```python
from build123d import *

# Parameters (mm, degrees)
BOSS_EXTRUDE1_DEPTH = 44.704
CUT_EXTRUDE1_DEPTH  = 55.481223747
CUT_EXTRUDE2_DEPTH  = 55.481223747


with BuildPart() as part:
    # Sketch1 → Boss-Extrude1 (new body)
    with BuildSketch(Plane(origin=(0, 0, 0), x_dir=(1, 0, 0), z_dir=(0, 1, 0))):
        with BuildLine():
            Line((19.604538786, -1.778), (-19.604538786, -1.778))
            ThreePointArc((-19.604538786, -1.778), (0, -19.685), (19.604538786, -1.778))
        make_face()
        with BuildLine():
            Line((-24.13, 1.778), (-24.13, -1.778))
            Line((-24.13, -1.778), (-19.604538786, -1.778))
            ThreePointArc((-19.604538786, -1.778), (-19.685, 0), (-19.604538786, 1.778))
            Line((-19.604538786, 1.778), (-24.13, 1.778))
        make_face()
        with BuildLine():
            ThreePointArc((19.685, 0), (19.664874408, -0.889909828), (19.604538786, -1.778))
            Line((19.604538786, -1.778), (24.13, -1.778))
            Line((24.13, -1.778), (24.13, 1.778))
            Line((24.13, 1.778), (19.604538786, 1.778))
            ThreePointArc((19.604538786, 1.778), (19.664874408, 0.889909828), (19.685, 0))
        make_face()
        with BuildLine():
            ThreePointArc((-19.604538786, 1.778), (-19.685, 0), (-19.604538786, -1.778))
            Line((-19.604538786, -1.778), (19.604538786, -1.778))
            ThreePointArc((19.604538786, -1.778), (19.664874408, -0.889909828), (19.685, 0))
            ThreePointArc((19.685, 0), (19.664874408, 0.889909828), (19.604538786, 1.778))
            Line((19.604538786, 1.778), (-19.604538786, 1.778))
        make_face()
        with BuildLine():
            ThreePointArc((-10.145068686, 16.869404446), (-16.679250829, 10.454750919), (-19.604538786, 1.778))
            Line((-19.604538786, 1.778), (19.604538786, 1.778))
            ThreePointArc((19.604538786, 1.778), (16.371852187, 10.929852742), (9.158931314, 17.424500056))
            Line((9.158931314, 17.424500056), (9.158931314, 11.559229776))
            Line((9.158931314, 11.559229776), (-10.145068686, 11.559229776))
            Line((-10.145068686, 11.559229776), (-10.145068686, 16.869404446))
        make_face()
    extrude(amount=BOSS_EXTRUDE1_DEPTH)

    # Sketch3 → Cut-Extrude1 (cut, through all)
    with BuildSketch(Plane(origin=(0, 44.704, 0), x_dir=(1, 0, 0), z_dir=(0, 1, 0))):
        with BuildLine():
            Line((-18.40799177, 0.508), (-18.40799177, -0.508))
            ThreePointArc((-18.40799177, -0.508), (0, -18.415), (18.40799177, -0.508))
            Line((18.40799177, -0.508), (18.40799177, 0.508))
            ThreePointArc((18.40799177, 0.508), (16.176802096, 8.799051026), (10.428931314, 15.177273031))
            Line((10.428931314, 15.177273031), (10.428931314, 10.289229776))
            Line((10.428931314, 10.289229776), (-11.415068686, 10.289229776))
            Line((-11.415068686, 10.289229776), (-11.415068686, 14.450205254))
            ThreePointArc((-11.415068686, 14.450205254), (-16.460559091, 8.256041389), (-18.40799177, 0.508))
        make_face()
    extrude(amount=-CUT_EXTRUDE1_DEPTH, mode=Mode.SUBTRACT)

    # Sketch4 → Cut-Extrude2 (cut, through all)
    with BuildSketch(Plane(origin=(0, 44.704, 0), x_dir=(1, 0, 0), z_dir=(0, 1, 0))):
        Polygon((-11.415068686, 14.450205254), (-10.145068686, 15.334289128), (9.158931314, 15.334289128), (10.428931314, 15.177273031), (10.428931314, 10.289229776), (-11.415068686, 10.289229776), align=None)
    extrude(amount=-CUT_EXTRUDE2_DEPTH, mode=Mode.SUBTRACT)


solid = part.part
```
Input: part model. Units: mm. Frame: model coordinates. A direction names the side the tool comes from. Give positions to 0.01 mm unless a question says otherwise; leave off trailing zeros. Order: outer loops, then holes, each group sorted by start corner. A loop starts at its lowest first (then second) coordinate and runs counter-clockwise, first axis right, second up. Notation, with made-up numbers: (7, -34.5) - (12, -34.5) arc R30 ccw to (12, -5.5) - close; hole circle Ø4 at (45.25, 41.5). An arc over 180 degrees is marked (long way). One line per item, written item: value.
1. Draft query along Z for faces 1 (the face through (0, 44.704, 19)), 2 (the face through (22, 22, -1.778)), 3 (the face through (-10.789, 22.665, -14.886)), 4 (the face through (-16.41, 22.66, -8.36)). Return one class per face: released by +Z, released by -Z, zero draft, split by the parting line, or undercut.
Determined:
face 1: zero draft
face 2: released by -Z
face 3: undercut
face 4: undercut
2. Pin query (flat end, axial travel): pin 1 Ø2.5 at (x, y) = (-21, 33.5) entering from -Z; pin 2 Ø2.5 at (x, y) = (22, 21) entering from +Z; pin 3 Ø1.7 at (y, z) = (19, -16) entering from +X. Return the tip coordinate at first contact, or that it passes through.
Determined:
pin 1: z = -1.78
pin 2: z = 1.78
pin 3: x = 12.57
3. Cut plane D-D, the plane x = 0. Output: boundary loops of the cut face in (y, z) (3 decimals), and give its area (3 significant figures).
Determined:
outline: (0, 18.415) - (44.704, 18.415) - (44.704, 19.685) - (0, 19.685) - close
area: 56.8 mm2
4. Cut plane A-A, the plane z = 5.5. Output: boundary loops of the cut face in (x, y), and give its area (3 significant figures).
Determined:
outline: (-18.9, 0) - (-17.57, 0) - (-17.57, 44.7) - (-18.9, 44.7) - close; (17.57, 0) - (18.9, 0) - (18.9, 44.7) - (17.57, 44.7) - close
area: 119 mm2
5. Line query: probe 1 along X at (y, z) = (34.5, 0); probe 2 along Z at (x, y) = (-10.5, 42); probe 3 along Z at (x, y) = (20.5, 29). Output: solid intervals per line, ascending.
Determined:
probe 1: -24.13 to -18.41, 18.41 to 24.13
probe 2: -16.65 to -15.09, 15.13 to 16.65
probe 3: -1.78 to 1.78
6. Cut plane C-C, the plane z = -11.5. Output: boundary loops of the cut face in (x, y).
Determined:
outline: (-15.98, 0) - (-14.38, 0) - (-14.38, 44.7) - (-15.98, 44.7) - close; (14.38, 0) - (15.98, 0) - (15.98, 44.7) - (14.38, 44.7) - close
7. Reachability of faces 5 (the face through (-22, 22, 1.778)), 6 (the face through (22, 22, 1.778)), 7 (the face through (-10.145, 22, -16)), 8 (the face through (-0.4, 22.66, 18.41)), 9 (the face through (-22, 22, -1.778)) from +Z, -Z, +X, -X, +Y, -Y: full face, straight path, thin tool, end or side. Return the list, or none.
Determined:
face 5: +Z, -X, +Y, -Y
face 6: +Z, +X, +Y, -Y
face 7: -Z, +Y, -Y
face 8: +Y, -Y
face 9: -Z, -X, +Y, -Y
